The listing builds one solid part. Answer for the finished solid, in the listing's coordinates (mm). Face numbers are marked on the shaded views. A direction names the side the tool comes from. Coordinates: 2 decimals unless noted, no trailing zeros. Order: outer loops, then holes, each group sorted by start corner. A loop starts at its lowest first (then second) coordinate and runs counter-clockwise, first axis right, second up. Notation, with made-up numbers: (-4, 43) -> (21, 43) arc R19 ccw to (21, 73) -> close; hole circle Ø5 at (-38.75, 40). An arc over 180 degrees is marked (long way). Return JSON: item names as keys, results as strings.
```python
from build123d import *

# Parameters (mm, degrees)
PAD001_DEPTH = 3
FILLET001_R  = 0.6
FILLET002_R  = 0.5


with BuildPart() as part:
    # Sketch002 (on DatumPlane) → Pad001 (new body)
    with BuildSketch(Plane.YZ.offset(-3.381818)):
        Polygon((2, 12.172727), (17, 10.860397), (17, 7.99163), (13, 8.341585), (13, 9.841585), (3.5, 10.672727), (3.5, 1.672727), (13, 2.50387), (13, 4.00387), (17, 4.353824), (17, 1.485057), (2, 0.172727), (2, 3.672727), (0.5, 3.672727), (0.5, 8.672727), (2, 8.672727), align=None)
    extrude(amount=PAD001_DEPTH)

    # Fillet001
    fillet001_edges = [part.edges().sort_by_distance(p)[0] for p in [
        (-1.881818, 17, 4.353824),
        (-1.881818, 17, 10.860397),
        (-1.881818, 17, 7.99163),
        (-1.881818, 17, 1.485057),
        (-1.881818, 13, 8.341585),
        (-1.881818, 13, 4.00387),
        (-1.881818, 13, 2.50387),
        (-1.881818, 13, 9.841585),
    ]]
    fillet(fillet001_edges, radius=FILLET001_R)

    # Fillet002
    fillet002_edges = [part.edges().sort_by_distance(p)[0] for p in [
        (-1.881818, 2, 0.172727),
        (-1.881818, 3.5, 1.672727),
        (-1.881818, 3.5, 10.672727),
        (-1.881818, 2, 12.172727),
    ]]
    fillet(fillet002_edges, radius=FILLET002_R)


solid = part.part
```
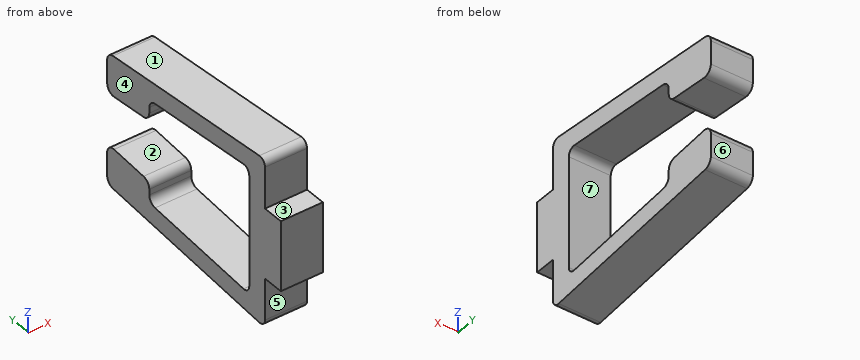
Item 1: Find the intervals of material crossed by probe 1 along Y at (x, z) = (-2.75, 9.25); probe 2 along Y at (x, z) = (-3.1, 5); probe 3 along Z at (x, y) = (-3.15, 8.5), in increasing order.
Answer list:
{"probe 1": "2 to 3.5, 13 to 17", "probe 2": "0.5 to 3.5", "probe 3": "0.74 to 2.11, 10.24 to 11.6"}
Item 2: The part is cut by section C-C on z = 5.25. Determine the outline of the cut face in (x, y).
Answer list:
{"outline": "(-3.38, 0.5) -> (-0.38, 0.5) -> (-0.38, 3.5) -> (-3.38, 3.5) -> close"}
Item 3: Flat-ended cylindrical pins translate along their axes: pin 1 (6 mm diameter, centred on y = 8, z = 3, fed in from +X); pin 2 (1.6 mm diameter, centred on x = -1, y = 1.5, fed in from -Z). Find the tip coordinate at first contact, or state that the pin passes through.
Answer list:
{"pin 1": "x = -0.38", "pin 2": "z = 0.26"}
Item 4: The part is cut by section A-A on y = 6. Determine the outline of the cut face in (x, z), plus the area to 3 significant figures.
Answer list:
{"outline": "(-3.38, 0.52) -> (-0.38, 0.52) -> (-0.38, 1.89) -> (-3.38, 1.89) -> close; (-3.38, 10.45) -> (-0.38, 10.45) -> (-0.38, 11.82) -> (-3.38, 11.82) -> close", "area": "8.21 mm2"}
Item 5: Determine the mould class of the marked faces 4, 5, 6 and 7 for opening direction Y: pulls with the +Y half, pulls with the -Y half, needs draft (parallel to the pull), parting line crosses it, or undercut.
Answer list:
{"face 4": "needs draft", "face 5": "pulls with the -Y half", "face 6": "pulls with the +Y half", "face 7": "undercut"}
Item 6: The part is cut by section B-B on x = -1.3. Determine the outline of the cut face in (y, z), plus the area to 3 significant figures.
Answer list:
{"outline": "(0.5, 3.67) -> (2, 3.67) -> (2, 0.72) arc R0.5 ccw to (2.54, 0.22) -> (16.45, 1.44) arc R0.6 ccw to (17, 2.03) -> (17, 3.7) arc R0.6 ccw to (16.35, 4.3) -> (13.55, 4.05) arc R0.6 ccw to (13, 3.45) -> (13, 3.05) arc R0.6 cw to (12.45, 2.46) -> (4.04, 1.72) arc R0.5 cw to (3.5, 2.22) -> (3.5, 10.13) arc R0.5 cw to (4.04, 10.63) -> (12.45, 9.89) arc R0.6 cw to (13, 9.29) -> (13, 8.89) arc R0.6 ccw to (13.55, 8.29) -> (16.35, 8.05) arc R0.6 ccw to (17, 8.65) -> (17, 10.31) arc R0.6 ccw to (16.45, 10.91) -> (2.54, 12.13) arc R0.5 ccw to (2, 11.63) -> (2, 8.67) -> (0.5, 8.67) -> close", "area": "73.9 mm2"}
Item 7: Which of the six approach directions +Z, -Z, +X, -X, +Y, -Y give full straight-line access (tool end or side, diameter ignored) to the marked faces 1, 2 and 3?
Answer list:
{"face 1": "+Z, +X, -X, +Y", "face 2": "+X, -X", "face 3": "+Z, +X, -X, -Y"}
Item 8: The part is cut by section D-D on y = 14.75. Determine the outline of the cut face in (x, z).
Answer list:
{"outline": "(-3.38, 1.29) -> (-0.38, 1.29) -> (-0.38, 4.16) -> (-3.38, 4.16) -> close; (-3.38, 8.19) -> (-0.38, 8.19) -> (-0.38, 11.06) -> (-3.38, 11.06) -> close"}
